Read the model definition and answer for the solid it produces. Units are mm, in the model's axes. Face numbers are marked on the shaded views. Coordinates: 2 decimals unless noted, no trailing zeros. Write each loop counter-clockwise with the first axis right and the second up, starting at its lowest first coordinate (ties: lowest second). Pieces come first, ordered by that corner, then holes. Notation, with made-up numbers: (-35, -4.75) -> (-2, -4.75) arc R21 cw to (-2, 30.25) -> close; hole circle Ø1 at (-36, 71). An arc over 180 degrees is marked (long way). One line per item, written item: value. Start each with the question number.
1. Find section D-D, the plane y = 1.8. Write down the section's boundary in (x, z), and give its area (3 significant figures).
2. Find section C-C, the plane x = 11. Write down the section's boundary in (y, z), and give its area (4 significant figures).
3. Consider line 1 along X through (y, z) = (3.85, 0); line 2 along X through (y, z) = (1.75, 0); line 3 along Z through (x, y) = (7.5, 1.7). Determine where each line is inside the solid, lowest interval first.
4. Given P1, Ø0.8, axis at x = -10, y = 1.5, coming from the +Z side; P2, Ø2, axis at x = -7.5, y = 1.5, coming from the -Z side; P3, Ø1.8, axis at x = 20, z = 0, coming from the -Y side; P4, Ø1.5, axis at x = -15, z = 0.5, coming from the +Y side, each flat-ended and moving along its own axis, determine where each tip first touches the part or whether it passes through.
5. Find section A-A, the plane x = 0. Write down the section's boundary in (y, z), and give its area (3 significant figures).
6. For a pull along X with two mould halves and no side action, classify the marked faces 1, 2 and 3 as pulls with the +X half, pulls with the -X half, needs draft (parallel to the pull), parting line crosses it, or undercut.
7. Find section B-B, the plane y = 3.5. Write down the section's boundary in (x, z).
```python
from build123d import *
from build123d.topology import SkipClean

# Parameters (mm, degrees)
SKETCH_1_R      = 1
EXTRUDE_1_DEPTH = 3
EXTRUDE_2_DEPTH = 3
CHAMFER_1_SIZE  = 0.25
EXTRUDE_START   = 3
SKETCH_4_R      = 2.5
SKETCH_4_R_2    = 1
EXTRUDE_3_DEPTH = 3
CHAMFER_4_SIZE  = 0.25
CHAMFER_5_SIZE  = 0.25


with BuildPart() as part:
    # 草图1 → 凸台-拉伸1 (new body)
    with BuildSketch(Plane(origin=(0, 0, 0), x_dir=(1, 0, 0), z_dir=(0, 1, 0))):
        with BuildLine():
            Line((-18, 1.5), (-2, 1.5))
            ThreePointArc((-2, 1.5), (0, 2.5), (2, 1.5))
            Line((2, 1.5), (18, 1.5))
            ThreePointArc((18, 1.5), (22.5, 0), (18, -1.5))
            Line((18, -1.5), (2, -1.5))
            ThreePointArc((2, -1.5), (0, -2.5), (-2, -1.5))
            Line((-2, -1.5), (-18, -1.5))
            ThreePointArc((-18, -1.5), (-22.5, 0), (-18, 1.5))
        make_face()
        with Locations(Location((-20, 0, 0), (0, 0, 270))):
            Circle(SKETCH_1_R, mode=Mode.SUBTRACT)
        with Locations(Location((0, 0, 0), (0, 0, 270))):
            Circle(SKETCH_1_R, mode=Mode.SUBTRACT)
        with Locations(Location((20, 0, 0), (0, 0, 270))):
            Circle(SKETCH_1_R, mode=Mode.SUBTRACT)
    extrude(amount=EXTRUDE_1_DEPTH)

    # 草图2 → 凸台-拉伸2 (add)
    with BuildSketch(Plane(origin=(0, 0, 0), x_dir=(1, 0, 0), z_dir=(0, 1, 0))):
        with BuildLine():
            Line((4.5, 1.5), (0.578145, 2.432231))
            ThreePointArc((0.578145, 2.432231), (1.370756, 2.0907), (2, 1.5))
            Line((2, 1.5), (4.5, 1.5))
        make_face()
        with BuildLine():
            Line((4.5, -1.5), (0.578145, -2.432231))
            ThreePointArc((0.578145, -2.432231), (1.370756, -2.0907), (2, -1.5))
            Line((2, -1.5), (4.5, -1.5))
        make_face()
        with BuildLine():
            Line((15.5, 1.5), (19.421855, 2.432231))
            ThreePointArc((19.421855, 2.432231), (18.629244, 2.0907), (18, 1.5))
            Line((18, 1.5), (15.5, 1.5))
        make_face()
        with BuildLine():
            Line((15.5, -1.5), (19.421855, -2.432231))
            ThreePointArc((19.421855, -2.432231), (18.629244, -2.0907), (18, -1.5))
            Line((18, -1.5), (15.5, -1.5))
        make_face()
        with BuildLine():
            Line((-4.5, 1.5), (-2, 1.5))
            ThreePointArc((-2, 1.5), (-1.370756, 2.0907), (-0.578145, 2.432231))
            Line((-0.578145, 2.432231), (-4.5, 1.5))
        make_face()
        with BuildLine():
            Line((-15.5, -1.5), (-18, -1.5))
            ThreePointArc((-18, -1.5), (-18.629244, -2.0907), (-19.421855, -2.432231))
            Line((-19.421855, -2.432231), (-15.5, -1.5))
        make_face()
        with BuildLine():
            Line((-18, 1.5), (-15.5, 1.5))
            Line((-15.5, 1.5), (-19.421855, 2.432231))
            ThreePointArc((-19.421855, 2.432231), (-18.629244, 2.0907), (-18, 1.5))
        make_face()
        with BuildLine():
            Line((-2, -1.5), (-4.5, -1.5))
            Line((-4.5, -1.5), (-0.578145, -2.432231))
            ThreePointArc((-0.578145, -2.432231), (-1.370756, -2.0907), (-2, -1.5))
        make_face()
    extrude(amount=EXTRUDE_2_DEPTH)

    # 倒角1
    chamfer_1_edges = [part.edges().sort_by_distance(p)[0] for p in [
        (-10, 0, -1.5),
        (-2.539073, 0, -1.966116),
        (-20, 0, -1),
        (0, 0, -1),
        (20, 0, -1),
        (0, 0, -2.5),
        (2.539073, 0, -1.966116),
        (-22.5, 0, 0),
        (-17.460927, 0, -1.966116),
        (-10, 0, 1.5),
        (-17.460927, 0, 1.966116),
        (0, 0, 2.5),
        (-2.539073, 0, 1.966116),
        (10, 0, 1.5),
        (2.539073, 0, 1.966116),
        (22.5, 0, 0),
        (17.460927, 0, 1.966116),
        (10, 0, -1.5),
        (17.460927, 0, -1.966116),
    ]]
    chamfer(chamfer_1_edges, length=CHAMFER_1_SIZE)

    # 草图4 → 凸台-拉伸3 (add)
    # profile 1 of 2: a face of its own
    with SkipClean():  # the faces are left unmerged after this step: merging them gives an invalid solid
        with BuildSketch(Plane(origin=(0, 0, 0), x_dir=(1, 0, 0), z_dir=(0, 1, 0)).offset(EXTRUDE_START)):
            with Locations(Location((-20, 0, 0), (0, 0, 76.628849))):
                Circle(SKETCH_4_R)
            with Locations(Location((-20, 0, 0), (0, 0, 270))):
                Circle(SKETCH_4_R_2, mode=Mode.SUBTRACT)
        # profile 2 of 2: a face of its own
        with BuildSketch(Plane(origin=(0, 0, 0), x_dir=(1, 0, 0), z_dir=(0, 1, 0)).offset(EXTRUDE_START)):
            with Locations(Location((20, 0, 0), (0, 0, 103.371151))):
                Circle(SKETCH_4_R)
            with Locations(Location((20, 0, 0), (0, 0, 270))):
                Circle(SKETCH_4_R_2, mode=Mode.SUBTRACT)
        extrude(amount=EXTRUDE_3_DEPTH)

    # 倒角4
    chamfer_4_edges = [part.edges().sort_by_distance(p)[0] for p in [
        (-20.578145, 6, 2.432231),
        (-20, 6, -1),
        (20.578145, 6, 2.432231),
        (20, 6, -1),
    ]]
    chamfer(chamfer_4_edges, length=CHAMFER_4_SIZE)

    # 倒角5
    chamfer_5_edges = [part.edges().sort_by_distance(p)[0] for p in [
        (-10, 3, -1.5),
        (-2.539073, 3, -1.966116),
        (0, 3, -1),
        (0, 3, -2.5),
        (2.539073, 3, -1.966116),
        (-10, 3, 1.5),
        (0, 3, 2.5),
        (-2.539073, 3, 1.966116),
        (10, 3, 1.5),
        (2.539073, 3, 1.966116),
        (10, 3, -1.5),
    ]]
    chamfer(chamfer_5_edges, length=CHAMFER_5_SIZE)


solid = part.part
```
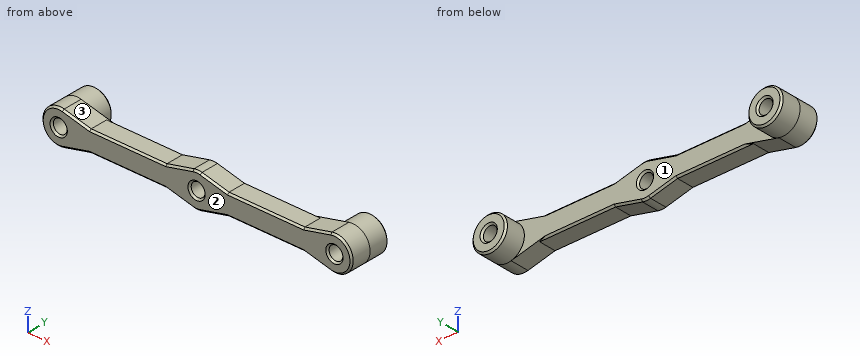
Answer block:
1. outline: (-19.42, -2.43) -> (-15.5, -1.5) -> (-4.5, -1.5) -> (-0.58, -2.43) arc R2.5 ccw to (0.58, -2.43) -> (4.5, -1.5) -> (15.5, -1.5) -> (19.42, -2.43) arc R2.5 ccw (long way) to (19.42, 2.43) -> (15.5, 1.5) -> (4.5, 1.5) -> (0.58, 2.43) arc R2.5 ccw to (-0.58, 2.43) -> (-4.5, 1.5) -> (-15.5, 1.5) -> (-19.42, 2.43) arc R2.5 ccw (long way) to start; hole circle Ø2 at (-20, 0); hole circle Ø2 at (0, 0); hole circle Ø2 at (20, 0)
1. area: 149 mm2
2. outline: (0, -1.25) -> (0.25, -1.5) -> (2.75, -1.5) -> (3, -1.25) -> (3, 1.25) -> (2.75, 1.5) -> (0.25, 1.5) -> (0, 1.25) -> close
2. area: 8.875 mm2
3. line 1: x = -22.5 to -21, -19 to -17.5, 17.5 to 19, 21 to 22.5
3. line 2: x = -22.5 to -21, -19 to -1, 1 to 19, 21 to 22.5
3. line 3: z = -1.5 to 1.5
4. P1: stops at z = 1.5
4. P2: stops at z = -1.5
4. P3: passes through
4. P4: stops at y = 3
5. outline: (0, -2.25) -> (0.25, -2.5) -> (2.75, -2.5) -> (3, -2.25) -> (3, -1.25) -> (2.75, -1) -> (0.25, -1) -> (0, -1.25) -> close; (0, 1.25) -> (0.25, 1) -> (2.75, 1) -> (3, 1.25) -> (3, 2.25) -> (2.75, 2.5) -> (0.25, 2.5) -> (0, 2.25) -> close
5. area: 8.75 mm2
6. face 1: undercut
6. face 2: needs draft
6. face 3: undercut
7. outline: circle Ø5 at (-20, 0); circle Ø5 at (20, 0); hole circle Ø2 at (-20, 0); hole circle Ø2 at (20, 0)
